Geometry: see drawing. Coordinates: mm, zero at the bounding-box minimum. Give positions to 0.01 mm unless a question says otherwise; leave off trailing zeros. Loops run counter-clockwise (first coordinate to the right, second up) from the corner with the lowest first, then second, coordinate; pieces in that order, holes last. Notation, with made-up numbers: M 1,7.5 L 51,7.5 A24 cw 51,20.5 Z; hole C 0,-31.5 d9. An arc over 180 degrees is marked long. Answer in a Markdown table with one row per item.
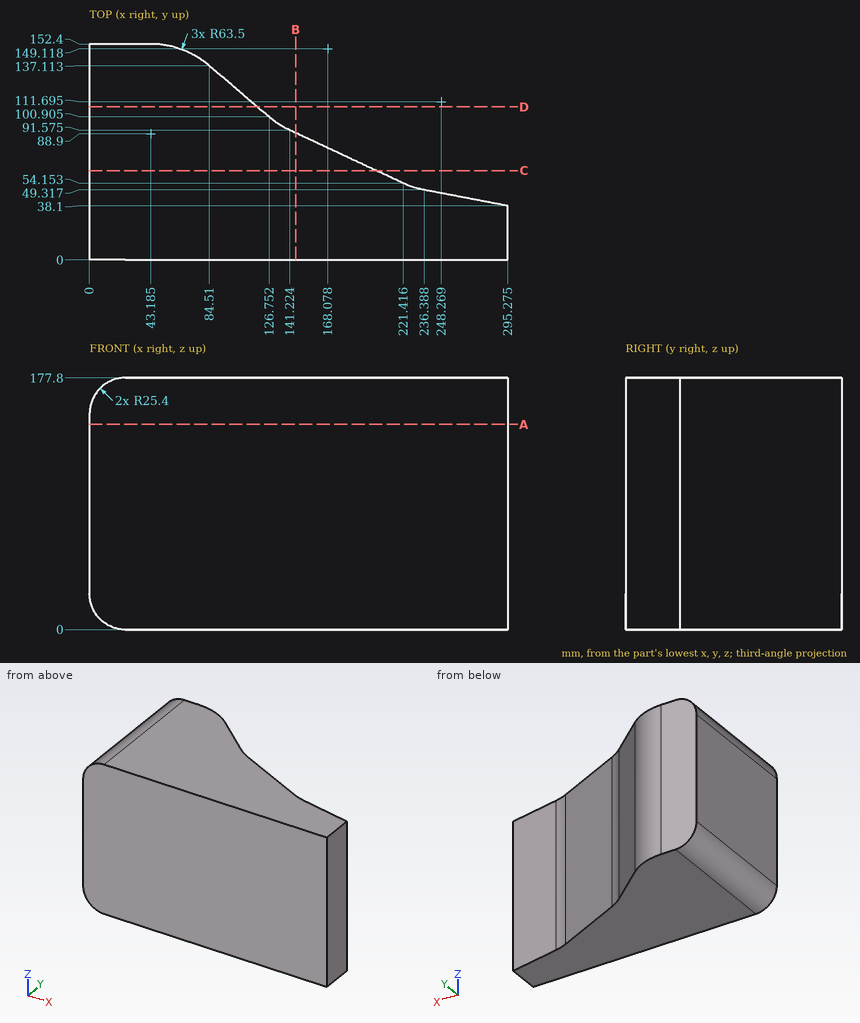
1) Section B-B, the plane x = 145.5. Return loops of the section in (y, z).
Reply:
| item | result |
|---|---|
| outline | M 0,0 L 89.58,0 L 89.58,177.8 L 0,177.8 Z |
2) Section A-A, the plane z = 145. Return loops of the section in (x, y) (1 decimal).
Reply:
| item | result |
|---|---|
| outline | M 0,0 L 295.3,0 L 295.3,38.1 L 236.4,49.3 A63.5 cw 221.4,54.2 L 141.2,91.6 A63.5 cw 126.8,100.9 L 84.5,137.1 A63.5 ccw 43.2,152.4 L 0,152.4 Z |
3) Section D-D, the plane y = 108. Return loops of the section in (x, z) (1 decimal).
Reply:
| item | result |
|---|---|
| outline | M 0,25.4 A25.4 ccw 25.4,0 L 118.5,0 L 118.5,177.8 L 25.4,177.8 A25.4 ccw 0,152.4 Z |
4) Section C-C, the plane y = 63. Return loops of the section in (x, z), then the cut area to 3 significant figures.
Reply:
| item | result |
|---|---|
| outline | M 0,25.4 A25.4 ccw 25.4,0 L 202.46,0 L 202.46,177.8 L 25.4,177.8 A25.4 ccw 0,152.4 Z |
| area | 35,700 mm² |
5) Pin query (flat end, axial travel): pin 1 Ø4 at (x, z) = (45.5, 61) entering from +Y; pin 2 Ø1 at (y, z) = (56.5, 156) entering from +X (1 decimal). Return the tip coordinate at first contact, or that it passes through.
Reply:
| item | result |
|---|---|
| pin 1 | stops at y = 152.4 |
| pin 2 | stops at x = 217.5 |
6) Material intervals for L1, parallel to X at y = 133.5, z = 83 (1 decimal); L2, parallel to X at y = 103.5, z = 65 (1 decimal); L3, parallel to Y at x = 66, z = 88, sorted ascending.
Reply:
| item | result |
|---|---|
| L1 | x = 0 to 88.7 |
| L2 | x = 0 to 123.7 |
| L3 | y = 0 to 148.16 |
